Drawing for the job (mm, zero at the part's lowest x, y, z). Coordinates: 2 decimals unless noted, no trailing zeros. Order: outer loops, then holes, each group sorted by start corner. A loop starts at its lowest first (then second) coordinate and runs counter-clockwise, first axis right, second up. Notation, with made-up numbers: (-23, 20.25) - (-13, 20.25) arc R29 ccw to (-13, 40.25) - close; hole circle Ø2 at (81, 61). An arc over 180 degrees is marked (long way). Put each result on its own line as item: value. Start each with the question number.
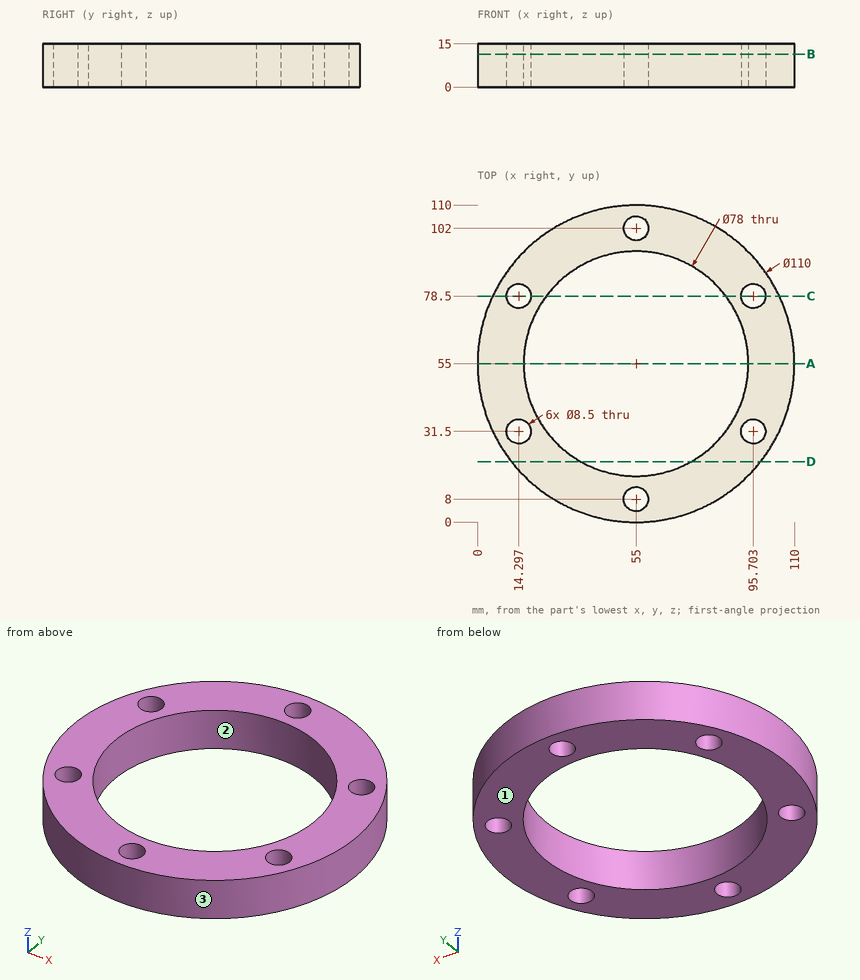
Item 1: Slice it at A-A, the plane y = 55. Give the cut face in (x, z), plus the area to 3 significant figures.
Item 2: Slice it at C-C, the plane y = 78.5. Give the cut face in (x, z) (1 decimal).
Item 3: Slice it at D-D, the plane y = 21. Give the cut face in (x, z) (3 decimals), plus the area to 3 significant figures.
Item 4: Pull direction Y, two halves, no side cores. Call the marked faces 1, 2 and 3: pulls with the +Y half, pulls with the -Y half, needs draft (parallel to the pull), parting line crosses it, or undercut.
Item 5: Wall check: line 1 along Y through (x, z) = (55, 6); line 2 along Y through (x, z) = (99.5, 8); line 3 along Y through (x, z) = (54, 12.75). Give the ranges that are in metal, low to high.
Item 6: Flat gauge pins, fed straight in: pin 1 Ø1 at (x, z) = (66, 5.5) entering from -Y; pin 2 Ø5 at (x, z) = (66, 4) entering from -Y; pin 3 Ø4 at (x, z) = (77.5, 4) entering from +Y; pin 4 Ø7 at (x, y) = (14.3, 78.5) entering from +Z. Where does each tip first touch, or does it go through?
Item 7: Slice it at B-B, the plane z = 11.5. Give the cut face in (x, y).
Here are the results:
1. outline: (0, 0) - (16, 0) - (16, 15) - (0, 15) - close; (94, 0) - (110, 0) - (110, 15) - (94, 15) - close
1. area: 480 mm^2
2. outline: (5.3, 0) - (10, 0) - (10, 15) - (5.3, 15) - close; (18.5, 0) - (23.9, 0) - (23.9, 15) - (18.5, 15) - close; (86.1, 0) - (91.5, 0) - (91.5, 15) - (86.1, 15) - close; (100, 0) - (104.7, 0) - (104.7, 15) - (100, 15) - close
3. outline: (11.768, 0) - (35.895, 0) - (35.895, 15) - (11.768, 15) - close; (74.105, 0) - (98.232, 0) - (98.232, 15) - (74.105, 15) - close
3. area: 724 mm^2
4. face 1: needs draft
4. face 2: undercut
4. face 3: parting line crosses it
5. line 1: y = 0 to 3.75, 12.25 to 16, 94 to 97.75, 106.25 to 110
5. line 2: y = 22.68 to 29.59, 33.41 to 76.59, 80.41 to 87.32
5. line 3: y = 0.01 to 3.87, 12.13 to 16.01, 93.99 to 97.87, 106.13 to 109.99
6. pin 1: stops at y = 1.01
6. pin 2: stops at y = 0.66
6. pin 3: stops at y = 106.04
6. pin 4: passes through
7. outline: circle Ø110 at (55, 55); hole circle Ø8.5 at (14.3, 31.5); hole circle Ø8.5 at (14.3, 78.5); hole circle Ø78 at (55, 55); hole circle Ø8.5 at (55, 8); hole circle Ø8.5 at (55, 102); hole circle Ø8.5 at (95.7, 31.5); hole circle Ø8.5 at (95.7, 78.5)
